from build123d import *

# Parameters (mm, degrees)
BOSS_EXTRUDE1_DEPTH = 152.4
SKETCH3_R           = 3.175
CUT_EXTRUDE1_DEPTH  = 159.876949241
BOSS_EXTRUDE2_START = -34.925
BOSS_EXTRUDE2_DEPTH = 12.7
BOSS_EXTRUDE3_DEPTH = 2.54
BOSS_EXTRUDE4_START = -12.7
BOSS_EXTRUDE4_DEPTH = 2.54
SKETCH7_R           = 1
CUT_EXTRUDE2_DEPTH  = 25.4
SKETCH8_W           = 36.576
SKETCH8_H           = 54.102
SKETCH8_W_2         = 26.416
SKETCH8_H_2         = 43.942
BOSS_EXTRUDE5_DEPTH = 18.415
SKETCH9_W           = 11.43
SKETCH9_H           = 8.89
CUT_EXTRUDE3_DEPTH  = 50.8
SKETCH10_R          = 3.175
SKETCH10_R_2        = 1.25
BOSS_EXTRUDE6_DEPTH = 6.35
SKETCH12_R          = 1.25
CUT_EXTRUDE4_DEPTH  = 161.317919845
SKETCH13_W          = 24.13
SKETCH13_H          = 16.166041667
CUT_EXTRUDE5_DEPTH  = 322.365846996
CUT_EXTRUDE6_START  = -69.85
CUT_EXTRUDE6_DEPTH  = 9.525
SKETCH15_R          = 1.25
CUT_EXTRUDE7_DEPTH  = 218.016479851


with BuildPart() as part:
    # Sketch2 → Boss-Extrude1 (new body)
    with BuildSketch(Plane.XY):
        with BuildLine():
            Line((-38.1, 6.35), (38.1, 6.35))
            ThreePointArc((38.1, 6.35), (44.45, 0), (38.1, -6.35))
            Line((38.1, -6.35), (-38.1, -6.35))
            ThreePointArc((-38.1, -6.35), (-44.45, 0), (-38.1, 6.35))
        make_face()
    extrude(amount=BOSS_EXTRUDE1_DEPTH)

    # Sketch3 → Cut-Extrude1 (cut, through all)
    with BuildSketch(Plane(origin=(0, 0, 0), x_dir=(-1, 0, 0), z_dir=(0, 0, -1))):
        with Locations((-38.1, 0)):
            Circle(SKETCH3_R)
        with Locations((38.1, 0)):
            Circle(SKETCH3_R)
    extrude(amount=-CUT_EXTRUDE1_DEPTH, mode=Mode.SUBTRACT)

    # Sketch5 → Boss-Extrude2 (add)
    with BuildSketch(Plane.XY.offset(152.4).offset(BOSS_EXTRUDE2_START)):
        with BuildLine():
            Line((26.040402296, 22.366781694), (32.390402296, 11.368259066))
            Line((32.390402296, 11.368259066), (43.388924924, 17.718259066))
            Line((43.388924924, 17.718259066), (44.45, 15.880423124))
            Line((44.45, 15.880423124), (44.45, 0))
            ThreePointArc((44.45, 0), (42.590128061, 4.490128061), (38.1, 6.35))
            Line((38.1, 6.35), (23.84069777, 6.35))
            Line((23.84069777, 6.35), (23.84069777, 21.096781694))
            Line((23.84069777, 21.096781694), (26.040402296, 22.366781694))
        make_face()
    extrude(amount=-BOSS_EXTRUDE2_DEPTH)

    # Sketch6 → Boss-Extrude3 (add)
    with BuildSketch(Plane.XY.offset(117.475)):
        with BuildLine():
            Line((23.84069777, 6.35), (38.1, 6.35))
            ThreePointArc((38.1, 6.35), (42.590128061, 4.490128061), (44.45, 0))
            Line((44.45, 0), (44.45, 15.880423124))
            Line((44.45, 15.880423124), (37.038924924, 28.716781694))
            Line((37.038924924, 28.716781694), (23.84069777, 21.096781694))
            Line((23.84069777, 21.096781694), (23.84069777, 6.35))
        make_face()
    extrude(amount=BOSS_EXTRUDE3_DEPTH)

    # Sketch6<2> → Boss-Extrude4 (add)
    with BuildSketch(Plane.XY.offset(117.475).offset(BOSS_EXTRUDE4_START)):
        with BuildLine():
            Line((23.84069777, 6.35), (38.1, 6.35))
            ThreePointArc((38.1, 6.35), (42.590128061, 4.490128061), (44.45, 0))
            Line((44.45, 0), (44.45, 15.880423124))
            Line((44.45, 15.880423124), (37.038924924, 28.716781694))
            Line((37.038924924, 28.716781694), (23.84069777, 21.096781694))
            Line((23.84069777, 21.096781694), (23.84069777, 6.35))
        make_face()
    extrude(amount=-BOSS_EXTRUDE4_DEPTH)

    # Sketch7 → Cut-Extrude2 (cut)
    with BuildSketch(Plane(origin=(-48.529047444, -83.623680275, 120.015), x_dir=(1, 0, 0), z_dir=(0, 0, 1))):
        with Locations(Location((85.148711054, 100.366643867, 0), (0, 0, 180))):
            Circle(SKETCH7_R)
        with Locations(Location((81.338711054, 106.965757444, 0), (0, 0, 180))):
            Circle(SKETCH7_R)
    extrude(amount=-CUT_EXTRUDE2_DEPTH, mode=Mode.SUBTRACT)

    # Sketch8 → Boss-Extrude5 (add)
    with BuildSketch(Plane(origin=(0, 6.35, 0), x_dir=(1, 0, 0), z_dir=(0, 1, 0))):
        with Locations((10.63269777, -73.914)):
            Rectangle(SKETCH8_W, SKETCH8_H)
        with Locations((10.63269777, -73.914)):
            Rectangle(SKETCH8_W_2, SKETCH8_H_2, mode=Mode.SUBTRACT)
    extrude(amount=BOSS_EXTRUDE5_DEPTH)

    # Sketch9 → Cut-Extrude3 (cut)
    with BuildSketch(Plane(origin=(28.92069777, -83.623680275, -42.409589959), x_dir=(0, 0, -1), z_dir=(1, 0, 0))):
        with Locations((-137.659589959, 103.943680275)):
            Rectangle(SKETCH9_W, SKETCH9_H)
    extrude(amount=-CUT_EXTRUDE3_DEPTH, mode=Mode.SUBTRACT)

    # Sketch10 → Boss-Extrude6 (add)
    with BuildSketch(Plane(origin=(0, 6.35, 0), x_dir=(1, 0, 0), z_dir=(0, 1, 0))):
        with Locations(Location((31.765, -8.938, 0), (0, 0, 270))):
            Circle(SKETCH10_R)
        with Locations(Location((31.765, -8.938, 0), (0, 0, 270))):
            Circle(SKETCH10_R_2, mode=Mode.SUBTRACT)
    boss_extrude6 = extrude(amount=BOSS_EXTRUDE6_DEPTH)

    # Sketch12 → Cut-Extrude4 (cut, through all)
    with BuildSketch(Plane(origin=(0, 6.35, 0), x_dir=(1, 0, 0), z_dir=(0, 1, 0))):
        with Locations(Location((31.765, -8.938, 0), (0, 0, 270))):
            Circle(SKETCH12_R)
    cut_extrude4 = extrude(amount=-CUT_EXTRUDE4_DEPTH, mode=Mode.SUBTRACT)

    # Sketch-Pattern1: Boss-Extrude6, Cut-Extrude4 at 7 more places
    with Locations((0, 0, 31.4), (-14, 0, 31.4), (-14, 0, 0), (-45.840002, 0, 14.477001), (-63.489998, 0, 14.477001), (-63.489998, 0, 107.627), (-45.840002, 0, 107.627)):
        add(boss_extrude6)
        add(cut_extrude4, mode=Mode.SUBTRACT)

    # Sketch13 → Cut-Extrude5 (cut, through all)
    with BuildSketch(Plane(origin=(55.039702575, 6.35, 304.758156205), x_dir=(-1, 0, 0), z_dir=(0, 1, 0))):
        with Locations((55.039702575, -296.675135372)):
            Rectangle(SKETCH13_W, SKETCH13_H)
    extrude(amount=-CUT_EXTRUDE5_DEPTH, mode=Mode.SUBTRACT)

    # Sketch14 → Cut-Extrude6 (cut)
    with BuildSketch(Plane(origin=(-48.529047444, -83.623680275, 0), x_dir=(-1, 0, 0), z_dir=(0, 0, -1)).offset(CUT_EXTRUDE6_START)):
        with BuildLine():
            Line((-74.909745214, 99.498680275), (-74.909745214, 77.273680275))
            Line((-74.909745214, 77.273680275), (-77.449745214, 77.273680275))
            Line((-77.449745214, 77.273680275), (-77.449745214, 108.388680275))
            Line((-77.449745214, 108.388680275), (-72.369745214, 108.388680275))
            Line((-72.369745214, 108.388680275), (-72.369745214, 105.848680275))
            ThreePointArc((-72.369745214, 105.848680275), (-74.251194346, 102.918259928), (-74.909745214, 99.498680275))
        make_face()
        with BuildLine():
            Line((-45.953745214, 105.848680275), (-45.953745214, 108.388680275))
            Line((-45.953745214, 108.388680275), (-40.873745214, 108.388680275))
            Line((-40.873745214, 108.388680275), (-40.873745214, 77.273680275))
            Line((-40.873745214, 77.273680275), (-43.413745214, 77.273680275))
            Line((-43.413745214, 77.273680275), (-43.413745214, 99.498680275))
            ThreePointArc((-43.413745214, 99.498680275), (-44.072296083, 102.918259928), (-45.953745214, 105.848680275))
        make_face()
    extrude(amount=-CUT_EXTRUDE6_DEPTH, mode=Mode.SUBTRACT)

    # Sketch15 → Cut-Extrude7 (cut, through all)
    with BuildSketch(Plane(origin=(-48.529047444, 6.35, -42.409589959), x_dir=(1, 0, 0), z_dir=(0, 1, 0))):
        with Locations(Location((57.927047444, -179.950589959, 0), (0, 0, 270))):
            Circle(SKETCH15_R)
        with Locations(Location((48.529047444, -179.950589959, 0), (0, 0, 270))):
            Circle(SKETCH15_R)
        with Locations(Location((39.131047444, -179.950589959, 0), (0, 0, 270))):
            Circle(SKETCH15_R)
    extrude(amount=-CUT_EXTRUDE7_DEPTH, mode=Mode.SUBTRACT)


solid = part.part
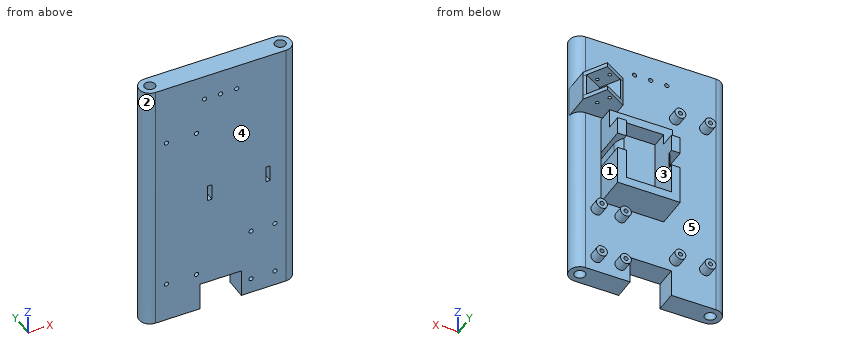
The listing builds one solid part. Answer for the finished solid, in the listing's coordinates (mm). Face numbers are marked on the shaded views. A direction names the side the tool comes from. Round coordinates to 2 decimals unless told otherwise and drop trailing zeros. Write each loop counter-clockwise with the first axis right and the second up, starting at its lowest first coordinate (ties: lowest second). Pieces come first, ordered by that corner, then holes. Notation, with made-up numbers: (43.5, 63.25) - (75.5, 63.25) arc R26 cw to (75.5, 84.25) - close; hole circle Ø9 at (20, 14.5). An arc over 180 degrees is marked (long way). Use one line per item in the form item = value. Start each with the question number.
Item 1: Determine the mould class of the marked faces 1, 2 and 3 for opening direction X: +X half, -X half, draft (parallel to the pull), parting line (faces both ways), or undercut.
Item 2: Find the intervals of material crossed by line 1 (X direction, y = 2, z = 33); line 2 (X direction, y = 12, z = 116.5); line 3 (X direction, y = 10, z = 90), in increasing order. Write a range as [from, to].
Item 3: A cutting plane is placed at B-B (z = 133). Write down the section's boundary in (x, y) (3 decimals).
Item 4: A tool of negligible diameter and unlimited length cuts with its end or side. For the marked faces 4 and 5, from which of +Z, -Z, +X, -X, +Y, -Y can it reach the whole face along a straight path? Write none if from no direction.
Item 5: Flat-ended cylindrical pins translate along their axes: pin 1 Ø5.5 at (y, z) = (15.5, 75) entering from +X; pin 2 Ø5 at (x, y) = (-12, 13.5) entering from -Z; pin 3 Ø5 at (y, z) = (15, 23.5) entering from -X. Find the tip coordinate at first contact, or state that the pin passes through.
Item 6: A cutting plane is placed at A-A (z = 76.5). Give the number of separate pieces and of enclosed holes in the cut face, plus the area to 3 significant figures.
The answers:
q1.face_1 = +X half
q1.face_2 = -X half
q1.face_3 = undercut
q2.line_1 = [-44.13, -40.57], [-35.63, 35.63], [40.57, 44.13]
q2.line_2 = [-34.9, -32.97], [-30.48, -28.55], [-17.25, -15.32], [-12.83, -10.9], [23.84, 32.03], [33.48, 44.45]
q2.line_3 = [-7.66, -2.58], [23.84, 28.92]
q3.outline = (-38.1, -6.35) - (38.1, -6.35) arc R6.35 ccw to (38.1, 6.35) - (-38.1, 6.35) arc R6.35 ccw to start; hole circle Ø6.35 at (-38.1, 0); hole circle Ø6.35 at (38.1, 0)
q4.face_4 = +Z, -Z, +X, -X, -Y
q4.face_5 = +Y
q5.pin_1 = 26.38
q5.pin_2 = 20.24
q5.pin_3 = -34.9
q6.separate_pieces = 3
q6.enclosed_holes = 2
q6.area = 1,040 mm^2
